Part model, mm, in its own coordinate system. A direction names the side the tool comes from. Give positions to 0.01 mm unless a question says otherwise; leave off trailing zeros. Write each loop counter-clockwise with the first axis right and the second up, starting at its lowest first coordinate (ties: lowest second). Pieces come first, ordered by that corner, then holes. Notation, with made-up numbers: M 6,-16 L 28,-16 A8 cw 28,-2 Z; hole C -13,-11.75 d8. An arc over 180 degrees is marked long. Answer as CSV lines item,"result". Start each with the question number.
1) Slice it at D-D, the plane x = 10. Give the cut face in (y, z), plus the area to 3 significant figures.
2) Mould opens along X. For faces 1 (the flat face through (22.5, -13, 0)), 2 (the flat face through (-9, -11, 0)), 3 (the flat face through (35, 10, 0)) say: pulls with the +X half, pulls with the -X half, needs draft (parallel to the pull), parting line crosses it, or undercut.
3) Tool access for faces 4 (the flat face through (32.5, -12, 0)), 5 (the flat face through (2.5, -13, 0)), 6 (the flat face through (-10, 10, 0)), 7 (the flat face through (-7.5, -13, 0)): list every direction of +Z, -Z, +X, -X, +Y, -Y with a clear straight run to the whole face (end or side of a thin tool).
4) Slice it at C-C, the plane y = -9. Give the cut face in (x, z), plus the area to 3 significant figures.
5) Pin check, flat tips, straight feed: pin 1 Ø0.9 at (y, z) = (-13, 0) entering from -X; pin 2 Ø1.5 at (y, z) = (-5.5, 0.5) entering from -X; pin 3 Ø3 at (x, y) = (35, 4) entering from +Z. Stop position of each tip, or through.
6) Slice it at A-A, the plane x = 29. Give the cut face in (y, z).
7) Wall check: line 1 along X through (y, z) = (8, -1.35); line 2 along Y through (x, z) = (15, 1.25); line 3 along Y through (x, z) = (22, 0). Give the ranges that are in metal, low to high. Write a range as from..to.
8) Slice it at B-B, the plane z = -1.05. Give the cut face in (x, y), plus the area to 3 significant figures.
```python
from build123d import *

# Parameters (mm, degrees)
CROQUIS1_W              = 25
CROQUIS1_H              = 28
CROQUIS1_R              = 1.25
CROQUIS1_W_2            = 9.5
CROQUIS1_H_2            = 5
SALIENTE_EXTRUIR1_DEPTH = 1.5
CROQUIS4_W              = 20
CROQUIS4_H              = 3
CORTAR_EXTRUIR5_DEPTH   = 10


with BuildPart() as part:
    # Croquis1 → Saliente-Extruir1 (new, symmetric)
    # profile 1 of 2: a face of its own
    with BuildSketch(Plane.XY):
        Rectangle(CROQUIS1_W, CROQUIS1_H)
        with Locations((-10, 4)):
            Circle(CROQUIS1_R, mode=Mode.SUBTRACT)
        with Locations((10, 4)):
            Circle(CROQUIS1_R, mode=Mode.SUBTRACT)
        with Locations((0, 9.2)):
            Rectangle(CROQUIS1_W_2, CROQUIS1_H_2, mode=Mode.SUBTRACT)
    # profile 2 of 2: a face of its own
    with BuildSketch(Plane.XY):
        with Locations((25, 0)):
            Rectangle(CROQUIS1_W, CROQUIS1_H)
        with Locations((15, 4)):
            Circle(CROQUIS1_R, mode=Mode.SUBTRACT)
        with Locations((35, 4)):
            Circle(CROQUIS1_R, mode=Mode.SUBTRACT)
        with Locations((25, 9.2)):
            Rectangle(CROQUIS1_W_2, CROQUIS1_H_2, mode=Mode.SUBTRACT)
    extrude(amount=SALIENTE_EXTRUIR1_DEPTH, both=True)

    # Croquis4 → Cortar-Extruir5 (cut)
    with BuildSketch(Plane.XY.offset(1.5)):
        with BuildLine():
            Line((-10, 6.5), (-10, 14))
            Line((-10, 14), (-12.5, 14))
            Line((-12.5, 14), (-12.5, 4))
            ThreePointArc((-12.5, 4), (-11.767766953, 5.767766953), (-10, 6.5))
        make_face()
        with BuildLine():
            Line((-10, -11), (-10, 1.5))
            ThreePointArc((-10, 1.5), (-11.767766953, 2.232233047), (-12.5, 4))
            Line((-12.5, 4), (-12.5, -14))
            Line((-12.5, -14), (-7.5, -14))
            Line((-7.5, -14), (-7.5, -11))
            Line((-7.5, -11), (-10, -11))
        make_face()
        with Locations((12.5, -12.5)):
            Rectangle(CROQUIS4_W, CROQUIS4_H)
        with BuildLine():
            Line((37.5, -14), (37.5, 4))
            ThreePointArc((37.5, 4), (36.767766953, 2.232233047), (35, 1.5))
            Line((35, 1.5), (35, -11))
            Line((35, -11), (32.5, -11))
            Line((32.5, -11), (32.5, -14))
            Line((32.5, -14), (37.5, -14))
        make_face()
        with BuildLine():
            Line((37.5, 14), (35, 14))
            Line((35, 14), (35, 6.5))
            ThreePointArc((35, 6.5), (36.767766953, 5.767766953), (37.5, 4))
            Line((37.5, 4), (37.5, 14))
        make_face()
    extrude(amount=-CORTAR_EXTRUIR5_DEPTH, mode=Mode.SUBTRACT)


solid = part.part
```
Found:
1,outline,"M -11,-1.5 L 2.75,-1.5 L 2.75,1.5 L -11,1.5 Z; M 5.25,-1.5 L 14,-1.5 L 14,1.5 L 5.25,1.5 Z"
1,area,"67.5 mm²"
2,face 1,"undercut"
2,face 2,"needs draft"
2,face 3,"pulls with the +X half"
3,face 4,"+Z, -Z, +X, -Y"
3,face 5,"+Z, -Z, -Y"
3,face 6,"+Z, -Z, -X, +Y"
3,face 7,"+Z, -Z, -X, -Y"
4,outline,"M -10,-1.5 L 35,-1.5 L 35,1.5 L -10,1.5 Z"
4,area,"135 mm²"
5,pin 1,"x = -7.5"
5,pin 2,"x = -10"
5,pin 3,"z = 1.5"
6,outline,"M -14,-1.5 L 6.7,-1.5 L 6.7,1.5 L -14,1.5 Z; M 11.7,-1.5 L 14,-1.5 L 14,1.5 L 11.7,1.5 Z"
7,line 1,"-10..-4.75, 4.75..20.25, 29.75..35"
7,line 2,"-11..2.75, 5.25..14"
7,line 3,"-11..6.7, 11.7..14"
8,outline,"M -10,-11 L -7.5,-11 L -7.5,-14 L 2.5,-14 L 2.5,-11 L 22.5,-11 L 22.5,-14 L 32.5,-14 L 32.5,-11 L 35,-11 L 35,1.5 A2.5 ccw 35,6.5 L 35,14 L -10,14 L -10,6.5 A2.5 ccw -10,1.5 Z; hole C -10,4 d2.5; hole M -4.75,6.7 L 4.75,6.7 L 4.75,11.7 L -4.75,11.7 Z; hole C 10,4 d2.5; hole C 15,4 d2.5; hole M 20.25,6.7 L 29.75,6.7 L 29.75,11.7 L 20.25,11.7 Z; hole C 35,4 d2.5"
8,area,"1,090 mm²"
